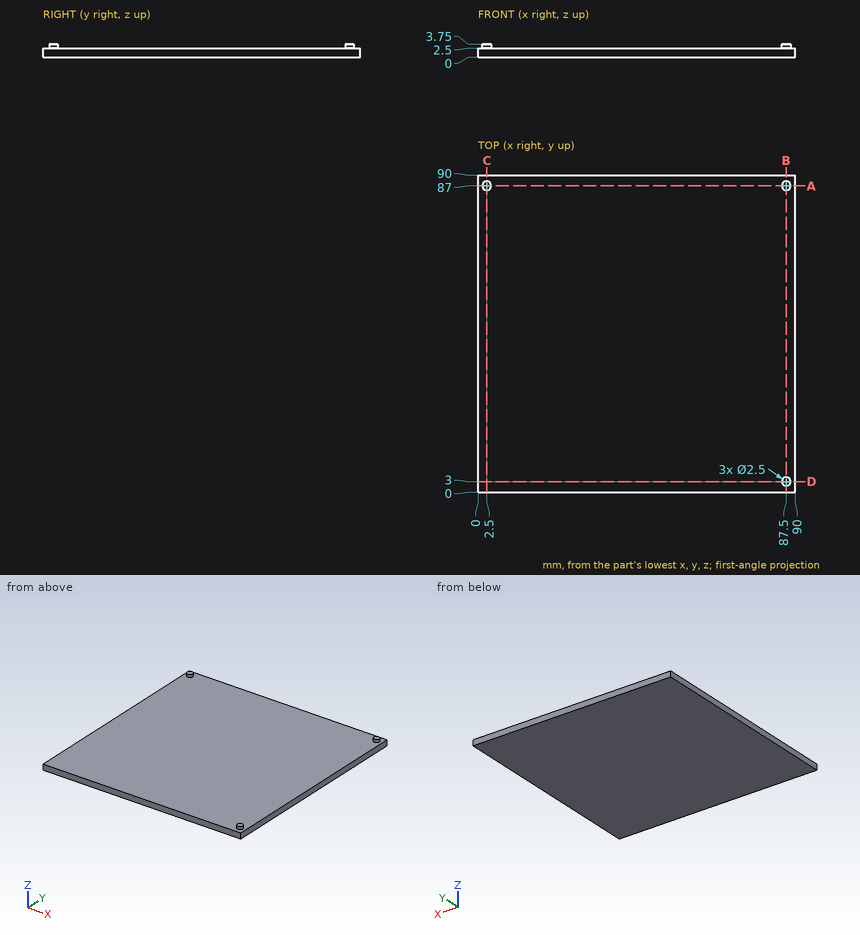
The drawing under review shows one solid part. Ordinate dimensions are in mm from its lowest x, y, z. Give positions to 0.01 mm unless a question says otherwise; leave off trailing zeros. Write each loop counter-clockwise with the first axis right and the second up, starting at its lowest first coordinate (ties: lowest second). Pieces come first, ordered by that corner, then holes. Notation, with made-up numbers: (-9, 24) - (44, 24) arc R31 ccw to (44, 59) - close; hole circle Ø1 at (66.5, 10.25). An arc over 180 degrees is marked (long way). Answer in a Markdown table with one row per item. Add a question column.
1. Wall thickness on line 1 along Z through (x, y) = (27.5, 53): over which ranges is the line inside the solid? List them lowest first. Write a range as [from, to].
2. We need section B-B on x = 87.5. Write out the cut boundary in (y, z), then the cut area to 3 significant figures.
3. We need section A-A on y = 87. Write out the cut boundary in (x, z), then the cut area to 3 significant figures.
4. We need section C-C on x = 2.5. Write out the cut boundary in (y, z), then the cut area to 3 significant figures.
5. We need section D-D on y = 3. Write out the cut boundary in (x, z).
Ans:
| question | item | result |
|---|---|---|
| 1 | line 1 | z = [0, 2.5] |
| 2 | outline | (0, 0) - (90, 0) - (90, 2.5) - (88.25, 2.5) - (88.25, 3.75) - (85.75, 3.75) - (85.75, 2.5) - (4.25, 2.5) - (4.25, 3.75) - (1.75, 3.75) - (1.75, 2.5) - (0, 2.5) - close |
| 2 | area | 231 mm^2 |
| 3 | outline | (0, 0) - (90, 0) - (90, 2.5) - (88.75, 2.5) - (88.75, 3.75) - (86.25, 3.75) - (86.25, 2.5) - (3.75, 2.5) - (3.75, 3.75) - (1.25, 3.75) - (1.25, 2.5) - (0, 2.5) - close |
| 3 | area | 231 mm^2 |
| 4 | outline | (0, 0) - (90, 0) - (90, 2.5) - (88.25, 2.5) - (88.25, 3.75) - (85.75, 3.75) - (85.75, 2.5) - (0, 2.5) - close |
| 4 | area | 228 mm^2 |
| 5 | outline | (0, 0) - (90, 0) - (90, 2.5) - (88.75, 2.5) - (88.75, 3.75) - (86.25, 3.75) - (86.25, 2.5) - (0, 2.5) - close |
